from build123d import *

# Parameters (mm, degrees)
F0_W     = 25
F0_H     = 30
F1_DEPTH = 6.5
F2_W     = 25
F2_H     = 2.1
F3_DEPTH = 25


with BuildPart() as f1:
    # F0 (on Front) → F1 (new body, symmetric)
    with BuildSketch(Plane.XZ):
        Rectangle(F0_W, F0_H)
    extrude(amount=F1_DEPTH, both=True)

    # F2 (on face) → F3 (cut)
    with BuildSketch(Plane(origin=(0, 0, -15), x_dir=(1, 0, 0), z_dir=(0, 0, -1))):
        with Locations((0, -2.55)):
            Rectangle(F2_W, F2_H)
    extrude(amount=-F3_DEPTH, mode=Mode.SUBTRACT)


solid = f1.part
CAD build for the part. Positions are in the model's coordinates, mm. A direction names the side the tool comes from. Round coordinates to 2 decimals unless told otherwise and drop trailing zeros. Order: outer loops, then holes, each group sorted by start corner. A loop starts at its lowest first (then second) coordinate and runs counter-clockwise, first axis right, second up. Notation, with made-up numbers: (-10.5, 3) -> (39.5, 3) arc R22 cw to (39.5, 36) -> close; hole circle Ø10 at (31, 80.5). An arc over 180 degrees is marked (long way). Write item = value, one per line. Start each with the question number.
(1) Cut at B-B, the plane x = 11.25. List the corners of the cut face in (y, z), then the cut area to 4 significant figures.
(2) Cut at C-C, the plane y = 2. List the corners of the cut face in (x, z).
(3) Probe line 1 (Y direction, x = -0.5, z = -9). List the from-to ranges inside material, lowest first. Write a range as [from, to].
(4) Cut at A-A, the plane z = -5. List the corners of the cut face in (x, y).
(5) Pull direction Y, two halves, no side cores. Call faces 1 (the flat face through (0, -3, -15)), 2 (the flat face through (0, 6.5, 0)), 3 (the flat face through (0, 1.5, -3)): released by +Y, released by -Y, zero draft, split by the parting line, or undercut.
(6) Pin check, flat tip, straight feed: P1, Ø1.7, axis at x = -4.5, y = 3, coming from the -Z side. Stop position of the tip, or through.
(7) Which spindle directions (+Z, -Z, +X, -X, +Y, -Y) get a long thin tool onto all of the face, cutting with end or side? Do faces 4 (the flat face through (12.5, 0, 0)), 5 (the flat face through (0, 3.6, -3)). Say none if no direction does.
Model answer:
q1.outline = (-6.5, -15) -> (1.5, -15) -> (1.5, 10) -> (3.6, 10) -> (3.6, -15) -> (6.5, -15) -> (6.5, 15) -> (-6.5, 15) -> close
q1.area = 337.5 mm2
q2.outline = (-12.5, 10) -> (12.5, 10) -> (12.5, 15) -> (-12.5, 15) -> close
q3.line_1 = [-6.5, 1.5], [3.6, 6.5]
q4.outline = (-12.5, -6.5) -> (12.5, -6.5) -> (12.5, 1.5) -> (-12.5, 1.5) -> close; (-12.5, 3.6) -> (12.5, 3.6) -> (12.5, 6.5) -> (-12.5, 6.5) -> close
q5.face_1 = zero draft
q5.face_2 = released by +Y
q5.face_3 = undercut
q6.P1 = -15
q7.face_4 = +Z, -Z, +X, +Y, -Y
q7.face_5 = -Z, +X, -X
